```python
from build123d import *

# Parameters (mm, degrees)
SKETCH1_W           = 190.5
SKETCH1_H           = 133.35
BOSS_EXTRUDE1_DEPTH = 3.175
SKETCH3_R           = 21.59
CUT_EXTRUDE2_DEPTH  = 117.310785183
SKETCH4_R           = 1.5875
CUT_EXTRUDE3_DEPTH  = 3.175
SKETCH9_R           = 2
CUT_EXTRUDE5_DEPTH  = 10
SKETCH12_W          = 98.425
SKETCH12_H          = 133.35
CUT_EXTRUDE6_DEPTH  = 117.310785183
SKETCH13_R          = 3.175
CUT_EXTRUDE7_DEPTH  = 117.310785183
CUT_EXTRUDE8_DEPTH  = 117.310785183
BOSS_EXTRUDE2_DEPTH = 3.175
FILLET1_R           = 2.54
CUT_EXTRUDE9_DEPTH  = 117.310785325
FILLET2_R           = 2.54


with BuildPart() as part:
    # Sketch1 → Boss-Extrude1 (new body)
    with BuildSketch(Plane(origin=(0, 0, 0), x_dir=(1, 0, 0), z_dir=(0, 1, 0))):
        Rectangle(SKETCH1_W, SKETCH1_H)
    extrude(amount=BOSS_EXTRUDE1_DEPTH)

    # Sketch3 → Cut-Extrude2 (cut, through all)
    with BuildSketch(Plane(origin=(0, 3.175, 0), x_dir=(1, 0, 0), z_dir=(0, 1, 0))):
        with Locations(Location((-53.425, 0, 0), (0, 0, 270))):
            Circle(SKETCH3_R)
    extrude(amount=-CUT_EXTRUDE2_DEPTH, mode=Mode.SUBTRACT)

    # Sketch4 → Cut-Extrude3 (cut)
    with BuildSketch(Plane(origin=(0, 3.175, 0), x_dir=(1, 0, 0), z_dir=(0, 1, 0))):
        with Locations(Location((-70.425, 17, 0), (0, 0, 270))):
            Circle(SKETCH4_R)
        with Locations(Location((-36.425, 17, 0), (0, 0, 270))):
            Circle(SKETCH4_R)
        with Locations(Location((-70.425, -17, 0), (0, 0, 270))):
            Circle(SKETCH4_R)
        with Locations(Location((-36.425, -17, 0), (0, 0, 270))):
            Circle(SKETCH4_R)
    extrude(amount=-CUT_EXTRUDE3_DEPTH, mode=Mode.SUBTRACT)

    # Sketch9 → Cut-Extrude5 (cut)
    with BuildSketch(Plane(origin=(0, 3.175, 0), x_dir=(1, 0, 0), z_dir=(0, 1, 0))):
        with Locations(Location((-18.4365, 0, 0), (0, 0, 270))):
            Circle(SKETCH9_R)
    extrude(amount=-CUT_EXTRUDE5_DEPTH, mode=Mode.SUBTRACT)

    # Sketch12 → Cut-Extrude6 (cut, through all)
    with BuildSketch(Plane(origin=(0, 3.175, 0), x_dir=(1, 0, 0), z_dir=(0, 1, 0))):
        with Locations((46.0375, 0)):
            Rectangle(SKETCH12_W, SKETCH12_H)
    extrude(amount=-CUT_EXTRUDE6_DEPTH, mode=Mode.SUBTRACT)

    # Sketch13 → Cut-Extrude7 (cut, through all)
    with BuildSketch(Plane(origin=(0, 3.175, 0), x_dir=(1, 0, 0), z_dir=(0, 1, 0))):
        with Locations(Location((-63.5, -57.15, 0), (0, 0, 270))):
            Circle(SKETCH13_R)
        with Locations(Location((-31.75, -57.15, 0), (0, 0, 270))):
            Circle(SKETCH13_R)
        with Locations(Location((-85.725, -34.925, 0), (0, 0, 270))):
            Circle(SKETCH13_R)
        with Locations(Location((-85.725, 34.925, 0), (0, 0, 90))):
            Circle(SKETCH13_R)
        with Locations(Location((-31.75, 57.15, 0), (0, 0, 90))):
            Circle(SKETCH13_R)
        with Locations(Location((-63.5, 57.15, 0), (0, 0, 90))):
            Circle(SKETCH13_R)
    extrude(amount=-CUT_EXTRUDE7_DEPTH, mode=Mode.SUBTRACT)

    # Sketch14 → Cut-Extrude8 (cut, through all)
    with BuildSketch(Plane(origin=(0, 3.175, 0), x_dir=(1, 0, 0), z_dir=(0, 1, 0))):
        with BuildLine():
            Line((-28.5965, 10.795), (-34.727511532, 10.795))
            ThreePointArc((-34.727511532, 10.795), (-32.57066141, 5.587903184), (-31.835, 0))
            ThreePointArc((-31.835, 0), (-32.57066141, -5.587903184), (-34.727511532, -10.795))
            Line((-34.727511532, -10.795), (-28.5965, -10.795))
            ThreePointArc((-28.5965, -10.795), (-24.106371939, -8.935128061), (-22.2465, -4.445))
            Line((-22.2465, -4.445), (-22.2465, 4.445))
            ThreePointArc((-22.2465, 4.445), (-24.106371939, 8.935128061), (-28.5965, 10.795))
        make_face()
    extrude(amount=-CUT_EXTRUDE8_DEPTH, mode=Mode.SUBTRACT)

    # Sketch17 → Boss-Extrude2 (add)
    with BuildSketch(Plane(origin=(0, 3.175, 0), x_dir=(1, 0, 0), z_dir=(0, 1, 0))):
        with BuildLine():
            Line((-27.617916938, -2.569394862), (-29.842146395, -2.569394862))
            ThreePointArc((-29.842146395, -2.569394862), (-31.436748095, -3.132314839), (-32.324552038, -4.571563824))
            ThreePointArc((-32.324552038, -4.571563824), (-33.284202462, -7.776655742), (-34.727511532, -10.795))
            Line((-34.727511532, -10.795), (-28.5965, -10.795))
            ThreePointArc((-28.5965, -10.795), (-26.282004071, -10.358172465), (-24.285944537, -9.107790109))
            add(Edge.make_bspline(
                [(-24.285944537, -9.107790109), (-25.296427545, -8.702059101), (-27.426842977, -8.424005167), (-31.492325334, -5.200003891), (-29.562733021, -3.217728636), (-27.592836679, -2.82089378)],
                knots=[0.242965458, 0.242965458, 0.242965458, 0.242965458, 0.418906137, 0.719122828, 0.942603955, 0.942603955, 0.942603955, 0.942603955], degree=3))
            ThreePointArc((-27.592836679, -2.82089378), (-27.491543755, -2.683792533), (-27.617916938, -2.569394862))
        make_face()
        with BuildLine():
            Line((-34.727511532, 10.795), (-28.5965, 10.795))
            ThreePointArc((-28.5965, 10.795), (-26.282004071, 10.358172465), (-24.285944537, 9.107790109))
            add(Edge.make_bspline(
                [(-24.285944537, 9.107790109), (-25.296427545, 8.702059101), (-27.426842977, 8.424005167), (-31.492325334, 5.200003891), (-29.562733021, 3.217728636), (-27.592836679, 2.82089378)],
                knots=[0.242965458, 0.242965458, 0.242965458, 0.242965458, 0.418906137, 0.719122828, 0.942603955, 0.942603955, 0.942603955, 0.942603955], degree=3))
            ThreePointArc((-27.592836679, 2.82089378), (-27.491543755, 2.683792533), (-27.617916938, 2.569394862))
            Line((-27.617916938, 2.569394862), (-29.842146395, 2.569394862))
            ThreePointArc((-29.842146395, 2.569394862), (-31.436748095, 3.132314839), (-32.324552038, 4.571563824))
            ThreePointArc((-32.324552038, 4.571563824), (-33.284202462, 7.776655742), (-34.727511532, 10.795))
        make_face()
    extrude(amount=-BOSS_EXTRUDE2_DEPTH)

    # Fillet1
    fillet1_edges = [part.edges().sort_by_distance(p)[0] for p in [
        (-24.285944537, 1.5875, 9.107790109),
        (-24.285944537, 1.5875, -9.107790109),
    ]]
    fillet(fillet1_edges, radius=FILLET1_R)

    # Sketch20 → Cut-Extrude9 (cut, through all)
    with BuildSketch(Plane(origin=(0, 3.175, 0), x_dir=(1, 0, 0), z_dir=(0, 1, 0))):
        with BuildLine():
            Line((-32.388013842, -16.243224247), (-32.324552038, -4.571563824))
            ThreePointArc((-32.324552038, -4.571563824), (-31.835, 0), (-32.324552038, 4.571563824))
            Line((-32.324552038, 4.571563824), (-32.388013842, 16.243224247))
            ThreePointArc((-32.388013842, 16.243224247), (-30.609708534, 18.68014804), (-27.75696947, 17.698900276))
            ThreePointArc((-27.75696947, 17.698900276), (-22.2465, 0), (-27.75696947, -17.698900276))
            ThreePointArc((-27.75696947, -17.698900276), (-30.609708534, -18.68014804), (-32.388013842, -16.243224247))
        make_face()
    extrude(amount=-CUT_EXTRUDE9_DEPTH, mode=Mode.SUBTRACT)

    # Fillet2
    fillet2_edges = [part.edges().sort_by_distance(p)[0] for p in [
        (-32.324552038, 1.5875, 4.571563824),
        (-32.324552038, 1.5875, -4.571563824),
    ]]
    fillet(fillet2_edges, radius=FILLET2_R)


solid = part.part
```
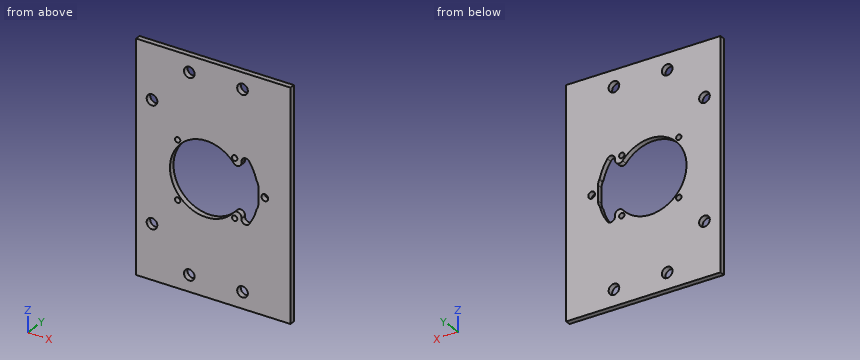
The listing builds one solid part. Answer for the finished solid, in the listing's coordinates (mm). Give positions to 0.01 mm unless a question says otherwise; leave off trailing zeros. Order: outer loops, then holes, each group sorted by start corner. A loop starts at its lowest first (then second) coordinate and runs counter-clockwise, first axis right, second up. Notation, with made-up numbers: (54, 84.25) -> (96, 84.25) arc R20 ccw to (96, 99.25) -> close; hole circle Ø6 at (-13.5, 32). An arc over 180 degrees is marked (long way). One line per item, written item: value.
1) A flat-ended cylindrical pin translates along its axis: P1, Ø2.5, axis at x = -36.425, z = 17, coming from the -Y side. Find the tip coordinate at first contact, or state that the pin passes through.
Reported:
P1: passes through
2) Find section B-B, the plane x = -55. Determine the outline of the cut face in (y, z) (3 decimals), plus the area to 3 significant figures.
Reported:
outline: (0, -66.675) -> (3.175, -66.675) -> (3.175, -21.532) -> (0, -21.532) -> close; (0, 21.532) -> (3.175, 21.532) -> (3.175, 66.675) -> (0, 66.675) -> close
area: 287 mm^2
3) Find section D-D, the plane y = 1.85. Count the separate pieces of the cut face and the enclosed holes in it, plus the area to 3 significant figures.
Reported:
separate pieces: 1
enclosed holes: 12
area: 10,200 mm^2
4) Find the intervals of material crossed by line 1 (X direction, y = 2.3, z = -57.15) (3 decimals); line 2 (Z direction, x = -35, y = 2.9) (3 decimals); line 3 (Z direction, x = -33, y = 0.4) (3 decimals), in increasing order.
Reported:
line 1: x = -95.25 to -66.675, -60.325 to -34.925, -28.575 to -3.175
line 2: z = -66.675 to -17.7, -16.3 to -12.952, 12.952 to 16.3, 17.7 to 66.675
line 3: z = -66.675 to -60.069, -54.231 to -13.833, 13.833 to 54.231, 60.069 to 66.675
5) Find section A-A, the plane z = 57.15. Determine the outline of the cut face in (x, y) (3 decimals), plus the area to 3 significant figures.
Reported:
outline: (-95.25, 0) -> (-66.675, 0) -> (-66.675, 3.175) -> (-95.25, 3.175) -> close; (-60.325, 0) -> (-34.925, 0) -> (-34.925, 3.175) -> (-60.325, 3.175) -> close; (-28.575, 0) -> (-3.175, 0) -> (-3.175, 3.175) -> (-28.575, 3.175) -> close
area: 252 mm^2
6) Find section C-C, the plane z = 10. Determine the outline of the cut face in (x, y) (3 decimals).
Reported:
outline: (-95.25, 0) -> (-72.559, 0) -> (-72.559, 3.175) -> (-95.25, 3.175) -> close; (-23.894, 0) -> (-3.175, 0) -> (-3.175, 3.175) -> (-23.894, 3.175) -> close
